```python
from build123d import *

# Parameters (mm, degrees)
F0_W     = 152.4
F0_H     = 228.6
F1_DEPTH = 5.08
F2_DEPTH = 2.54
F3_R     = 4.486697
F4_DEPTH = 1.27
F5_W     = 7.62
F5_H     = 2.54
F6_DEPTH = 5.08


with BuildPart() as f1:
    # F0 (on Top) → F1 (new body)
    with BuildSketch(Plane.XY):
        Rectangle(F0_W, F0_H)
        Polygon((69.85, -101.6), (-69.85, -101.6), (-69.85, 101.6), (-69.85, 107.95), (69.85, 107.95), (69.85, 101.6), align=None, mode=Mode.SUBTRACT)
    extrude(amount=F1_DEPTH)

    # F0 (on Top) → F2 (join)
    with BuildSketch(Plane.XY):
        Polygon((-69.85, 101.6), (-69.85, -101.6), (69.85, -101.6), (69.85, 101.6), (69.85, 107.95), (-69.85, 107.95), align=None)
    extrude(amount=F2_DEPTH)

    # F3 (on face) → F4 (cut)
    with BuildSketch(Plane.XY.offset(5.08)):
        with Locations((0, -107.710503)):
            Circle(F3_R)
    extrude(amount=-F4_DEPTH, mode=Mode.SUBTRACT)

    # F5 (on face) → F6 (cut)
    with BuildSketch(Plane.XZ.offset(114.3)):
        with Locations((-28.262435, 2.286)):
            Rectangle(F5_W, F5_H)
        with Locations((-11.677729, 2.286)):
            Rectangle(F5_W, F5_H)
    extrude(amount=-F6_DEPTH, mode=Mode.SUBTRACT)


solid = f1.part
```
Geometry check sheet. Reference: the model listing, model coordinates, mm. A direction names the side the tool comes from. Coordinates: 2 decimals unless noted, no trailing zeros. Write each loop counter-clockwise with the first axis right and the second up, starting at its lowest first coordinate (ties: lowest second). Pieces come first, ordered by that corner, then holes. Notation, with made-up numbers: M -21,80.5 L 2,80.5 A27 ccw 2,108.5 Z; hole C 50.25,88.5 d4. An arc over 180 degrees is marked long. Use one line per item in the form item = value. Start each with the question number.
1) Section check C-C on x = 0. Enter the section's corners in (y, z).
2) Go/stop test with flat-tipped pins: pin 1 Ø7 at (x, y) = (0, -107.71) entering from +Z; pin 2 Ø2.5 at (x, y) = (-10, -111) entering from -Z; pin 3 Ø2 at (x, z) = (-28, 2.5) entering from -Y. Record where each tip stops, or that it passes through.
3) Section check B-B on y = -12.5. Enter the section's corners in (x, z), and give its area (3 significant figures).
4) Section check A-A on x = -19.5. Enter the section's corners in (y, z), and give its area (3 significant figures).
5) Thickness scan on probe 1 along Y at (x, z) = (0, 4.6); probe 2 along X at (y, z) = (-40, 4.7); probe 3 along Y at (x, z) = (17, 2.8). Record the ranges inside material, lowest first. Write a range as from..to.
6) Release check for a two-part mould opening along Y. For faces 4 (the flat face through (-1, 114.3, 3)), 5 (the flat face through (-74, 9, 5.08)), 6 (the flat face through (0, -108, 3.81)) record: pulls with the +Y half, pulls with the -Y half, needs draft (parallel to the pull), parting line crosses it, or undercut.
7) Set-up check for faces 1 (the flat face through (-1, 5, 2.54)), 2 (the flat face through (-28, -112, 3.556)), 3 (the flat face through (-1, 2, 0)): record each of +Z, -Z, +X, -X, +Y, -Y from which the full face is reachable in a straight line by a thin tool's end or side.
Responses:
q1.outline = M -114.3,0 L 114.3,0 L 114.3,5.08 L 107.95,5.08 L 107.95,2.54 L -101.6,2.54 L -101.6,5.08 L -103.22,5.08 L -103.22,3.81 L -112.2,3.81 L -112.2,5.08 L -114.3,5.08 Z
q2.pin_1 = 3.81
q2.pin_2 = 0
q2.pin_3 = -109.22
q3.outline = M -76.2,0 L 76.2,0 L 76.2,5.08 L 69.85,5.08 L 69.85,2.54 L -69.85,2.54 L -69.85,5.08 L -76.2,5.08 Z
q3.area = 419 mm2
q4.outline = M -114.3,0 L 114.3,0 L 114.3,5.08 L 107.95,5.08 L 107.95,2.54 L -101.6,2.54 L -101.6,5.08 L -114.3,5.08 Z
q4.area = 629 mm2
q5.probe_1 = -114.3..-112.2, -103.22..-101.6, 107.95..114.3
q5.probe_2 = -76.2..-69.85, 69.85..76.2
q5.probe_3 = -114.3..-101.6, 107.95..114.3
q6.face_4 = pulls with the +Y half
q6.face_5 = needs draft
q6.face_6 = undercut
q7.face_1 = +Z
q7.face_2 = -Y
q7.face_3 = -Z, +X, -X, +Y, -Y
